Could you check a few things on this drawing? It's one solid part, dimensions in mm from its lowest x, y, z. Give positions to 0.01 mm unless a question says otherwise; leave off trailing zeros. Order: outer loops, then holes, each group sorted by start corner. A loop starts at its lowest first (then second) coordinate and runs counter-clockwise, first axis right, second up. Notation, with made-up numbers: M 31.5,42.25 L 35.5,42.25 A14 ccw 35.5,49.25 Z; hole C 84.25,83.25 d4. An arc over 180 degrees is marked long. Use one line per item in the form item = value. Start each with the question number.
1. Will these pins go through, and if not, where does the flat tip stop? P1, Ø10, axis at x = 125, y = 59.5, coming from the +Z side (1 decimal); P2, Ø3, axis at x = 49.5, z = 156.5, coming from the +Y side; P3, Ø2, axis at y = 11.5, z = 59, coming from the -X side (1 decimal); P4, Ø12.5, axis at x = 111.125, z = 111.125, coming from the +Y side.
2. I want a section at B-B, the plane y = 19. List the corners of the cut face in (x, z) for me (1 decimal), and give its area (3 significant figures).
3. I want a section at A-A, the plane z = 78.5. Count the separate pieces of the cut face and the enclosed holes in it, and give its area (3 significant figures).
4. I need wall thicknesses on L1, parallel to Y at x = 138.5, z = 89.5 (1 decimal); L2, parallel to Y at x = 63, z = 188; L3, parallel to Z at x = 116, y = 51 (1 decimal). Which ranges of each line are inside material? Lowest first, please.
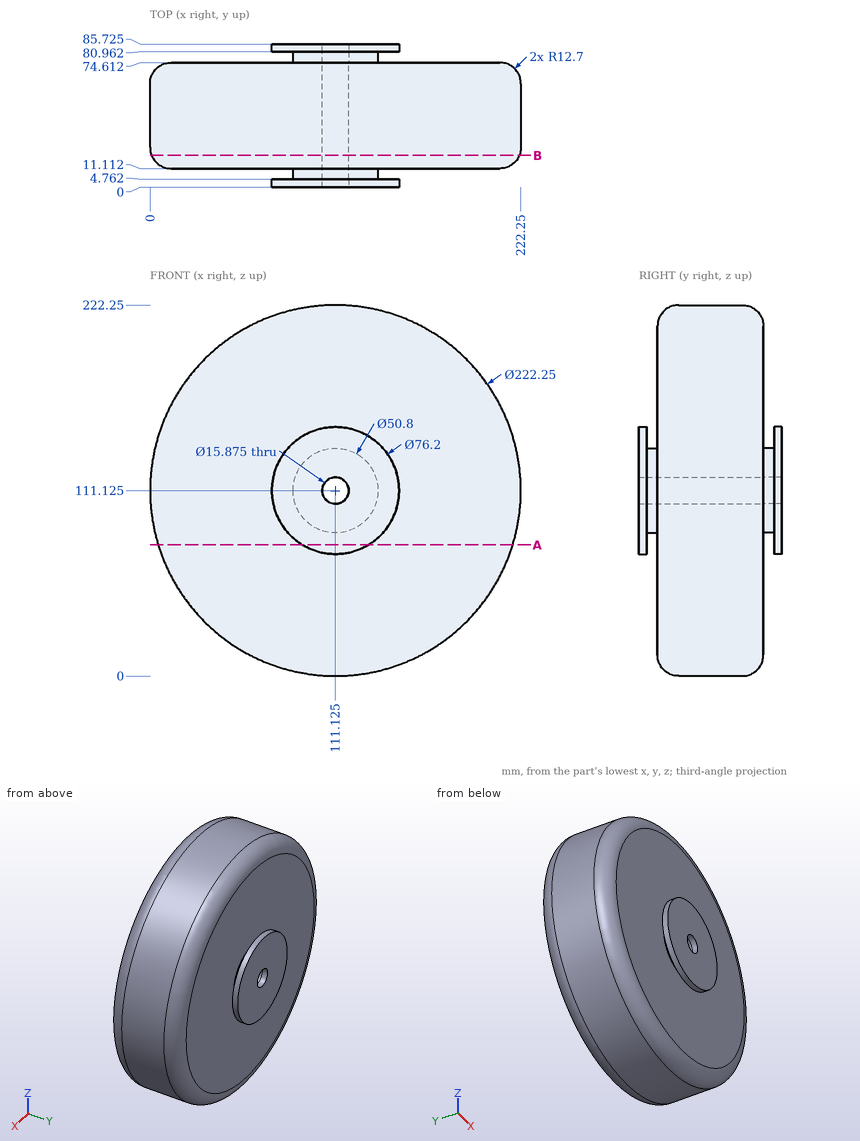
Check result:
q1.P1 = 221.9
q1.P2 = 74.61
q1.P3 = 20.8
q1.P4 = through
q2.outline = C 111.1,111.1 d220.4; hole C 111.1,111.1 d15.9
q2.area = 37,900 mm2
q3.separate_pieces = 3
q3.enclosed_holes = 0
q3.area = 13,700 mm2
q4.L1 = 0 to 4.8, 11.1 to 74.6, 81 to 85.7
q4.L2 = 11.11 to 74.61
q4.L3 = 0.1 to 104.9, 117.4 to 222.1
